Could you check a few things on this model? Use its own coordinates, in mm. Give positions to 0.01 mm unless a question says otherwise; leave off trailing zeros. Write each loop counter-clockwise with the first axis right and the second up, starting at its lowest first coordinate (ties: lowest second). Pieces come first, ordered by that corner, then holes. Notation, with made-up numbers: (47, 72) - (68, 72) arc R30 cw to (68, 110) - close; hole circle Ø9 at (-5.5, 50.5). An arc over 180 degrees is marked (long way). Write item = value, one per line.
Autodesk Fusion 360 part; units mm, degrees
sketch "phone" plane through (0, 0, 0) normal (0, 0, 1) x (1, 0, 0)
  line L0 (-42, -60) -> (-21, -60)
  arc A0 (-21, -60) -> (-12, -52) centre (-21, -50.9375) ccw
  line L1 (-12, -52) -> (-12, 53)
  arc A1 (-12, 53) -> (-20, 61) centre (-20, 53) ccw
  line L2 (-20, 61) -> (-42, 61)
  line L3 (-64, 61) -> (-42, 61)
  arc A2 (-64, 61) -> (-72, 53) centre (-64, 53) ccw
  line L4 (-72, -52) -> (-72, 53)
  arc A3 (-72, -52) -> (-63, -60) centre (-63, -50.9375) ccw
  line L5 (-42, -60) -> (-63, -60)
extrude "Extrude1" add sketch "phone" along normal blind 6.91
hole "Hole1" at (-64, 53, 6.91) direction (0, 0, -1) diameter 5 depth 40 tip angle 118
sketch "button" plane through (0, 0, 6.91) normal (0, 0, 1) x (-1, 0, 0)
  circle A0 centre (64, -53) radius 2.5
  arc A1 (21, 60) -> (12, 52) centre (21, 50.9375) ccw
  line L0 (12, 52) -> (12, -53)
  arc A2 (12, -53) -> (20, -61) centre (20, -53) ccw
  line L1 (20, -61) -> (64, -61)
  arc A3 (64, -61) -> (72, -53) centre (64, -53) ccw
  line L2 (72, -53) -> (72, 52)
  arc A4 (72, 52) -> (63, 60) centre (63, 50.9375) ccw
  line L3 (63, 60) -> (21, 60)
  line L4 (46.6846, 51.3855) -> (36.5241, 51.3855)
  line L5 (34.5241, 53.3855) -> (34.5241, 55.3855)
  line L6 (36.5241, 57.3855) -> (46.6846, 57.3855)
  line L7 (48.6846, 55.3855) -> (48.6846, 53.3855)
  arc A5 (46.6846, 51.3855) -> (48.6846, 53.3855) centre (46.6846, 53.3855) ccw
  arc A6 (48.6846, 55.3855) -> (46.6846, 57.3855) centre (46.6846, 55.3855) ccw
  arc A7 (34.5241, 53.3855) -> (36.5241, 51.3855) centre (36.5241, 53.3855) ccw
  arc A8 (36.5241, 57.3855) -> (34.5241, 55.3855) centre (36.5241, 55.3855) ccw
  dimension "d6" = 2
extrude "Extrude2" cut sketch "button" against normal blind 1 contours L4 L5 L6 L7 A5 A6 A7 A8
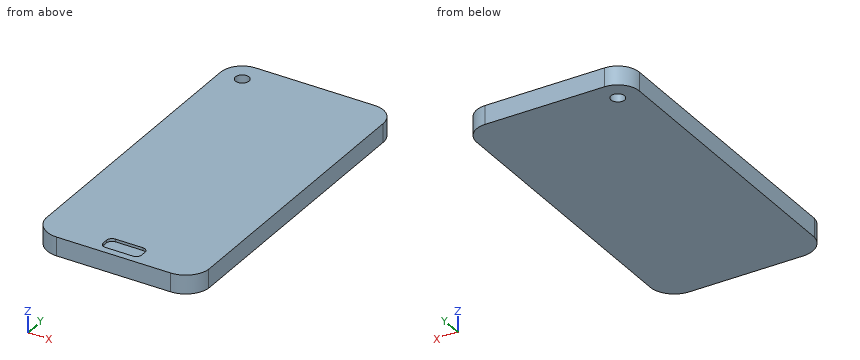
1. For pin 1 (0.8 mm diameter, centred on y = -54, z = 6.5, fed in from +X); pin 2 (1 mm diameter, centred on x = -28.5, y = 46.5, fed in from -Z); pin 3 (4 mm diameter, centred on x = -64, y = 53, fed in from +Z); pin 4 (5 mm diameter, centred on x = -42, y = -54, fed in from +Z), each with a flat end and sliding along its axis, tell me the tip position at first contact or that it passes through.
Filled sheet:
pin_1 = -12.34
pin_2 = 0
pin_3 = through
pin_4 = 5.91
2. I need wall thicknesses on line 1 (X direction, y = 53, z = 3); line 2 (X direction, y = 54, z = 1); line 3 (Y direction, x = -64, z = 2). Which ranges of each line are inside material? Lowest first, please.
Filled sheet:
line_1 = -72 to -66.5, -61.5 to -12
line_2 = -71.94 to -66.29, -61.71 to -12.06
line_3 = -59.94 to 50.5, 55.5 to 61
3. If we section it at A-A, the plane x = -16: Please give me the cut outline in (y, z), and give its area (3 significant figures).
Filled sheet:
outline = (-58.5, 0) - (59.93, 0) - (59.93, 6.91) - (-58.5, 6.91) - close
area = 818 mm2
